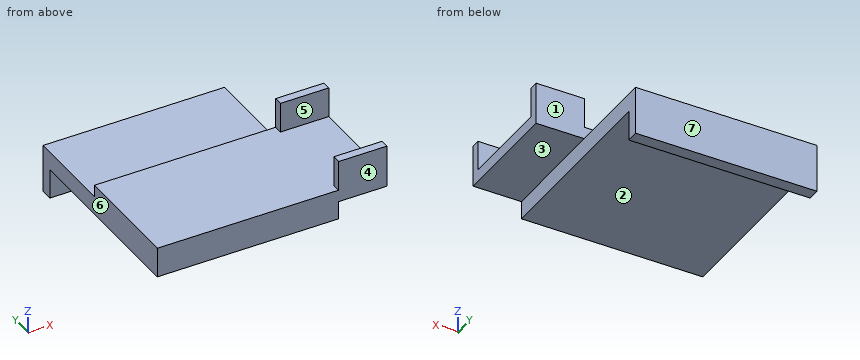
```python
from build123d import *

# Parameters (mm, degrees)
SKETCH2_W           = 50.8
SKETCH2_H           = 23.368
BOSS_EXTRUDE1_DEPTH = 2.54
SKETCH3_W           = 12.7
SKETCH3_H           = 1.778
BOSS_EXTRUDE2_DEPTH = 6.35
SKETCH4_W           = 2.54
SKETCH4_H           = 8.89
CUT_EXTRUDE1_DEPTH  = 24.368
BOSS_EXTRUDE3_DEPTH = 3.81
SKETCH10_W          = 38.1
SKETCH10_H          = 2.54
BOSS_EXTRUDE6_DEPTH = 6.35
SCALE1_SCALE        = 1.02


with BuildPart() as part:
    # Sketch2 → Boss-Extrude1 (new body)
    with BuildSketch(Plane.XY):
        Rectangle(SKETCH2_W, SKETCH2_H)
    extrude(amount=BOSS_EXTRUDE1_DEPTH)

    # Sketch3 → Boss-Extrude2 (add)
    with BuildSketch(Plane.XY.offset(2.54)):
        with Locations((19.05, 10.795)):
            Rectangle(SKETCH3_W, SKETCH3_H)
        with Locations((19.05, -10.795)):
            Rectangle(SKETCH3_W, SKETCH3_H)
    extrude(amount=BOSS_EXTRUDE2_DEPTH)

    # Sketch4 → Cut-Extrude1 (cut, through all)
    with BuildSketch(Plane(origin=(0, 11.684, 0), x_dir=(1, 0, 0), z_dir=(0, 1, 0))):
        with Locations((24.13, -4.445)):
            Rectangle(SKETCH4_W, SKETCH4_H)
    extrude(amount=-CUT_EXTRUDE1_DEPTH, mode=Mode.SUBTRACT)

    # Sketch5 → Boss-Extrude3 (add)
    with BuildSketch(Plane(origin=(0, 0, 0), x_dir=(-1, 0, 0), z_dir=(0, 0, -1))):
        Polygon((25.4, 11.684), (25.4, -11.684), (-12.7, -11.684), (-12.7, 11.684), (-12.7, 30.734), (25.4, 30.734), align=None)
    extrude(amount=BOSS_EXTRUDE3_DEPTH)

    # Sketch10 → Boss-Extrude6 (add)
    with BuildSketch(Plane(origin=(0, 0, -3.81), x_dir=(-1, 0, 0), z_dir=(0, 0, -1))):
        with Locations((6.35, 29.464)):
            Rectangle(SKETCH10_W, SKETCH10_H)
    extrude(amount=BOSS_EXTRUDE6_DEPTH)


with BuildPart() as part_1:
    # Scale1: scaled about (-4.313949838, 7.779949755, -1.122390582)
    add(part.part.scale(SCALE1_SCALE).moved(Location((0.086278997, -0.155598995, 0.022447812))))


solid = part_1.part
```
Can you work these out from the model? Positions are in its coordinate system, mm. Face numbers are marked on the shaded views. A direction names the side the tool comes from. Give positions to 0.01 mm unless a question says otherwise; leave off trailing zeros. Write each loop counter-clockwise with the first axis right and the second up, starting at its lowest first coordinate (ties: lowest second). Pieces come first, ordered by that corner, then holes. Notation, with made-up numbers: (80.5, -32) -> (129.5, -32) arc R30 cw to (129.5, 1) -> close; hole circle Ø4 at (76, 36.25). An arc over 180 degrees is marked (long way). One line per item, written item: value.
Q1. Imagine slicing it at B-B on x = 14.5. Please give me the cut outline in (y, z).
Results found:
outline: (-12.07, 0.02) -> (11.76, 0.02) -> (11.76, 9.09) -> (9.95, 9.09) -> (9.95, 2.61) -> (-10.26, 2.61) -> (-10.26, 9.09) -> (-12.07, 9.09) -> close
Q2. Please list where these lines run through material, in increasing order: line 1 (Z direction, x = 12.5, y = -2); line 2 (X direction, y = 29, z = -4.75); line 3 (Y direction, x = 9, z = -8.75). Write a range as [from, to].
Results found:
line 1: z = [-3.86, 2.61]
line 2: x = [-25.82, 13.04]
line 3: y = [28.6, 31.19]
Q3. We'd pull the mould along Y, two halves only. Please class the marked faces 5, 6 and 7: +Y half, -Y half, draft (parallel to the pull), parting line (faces both ways), or undercut.
Results found:
face 5: undercut
face 6: draft
face 7: +Y half
Q4. Which directions (+Z, -Z, +X, -X, +Y, -Y) give clear straight access to the entire face, cutting with the end or side of a thin tool? Please do the marked faces 1, 2, 3 and 4.
Results found:
face 1: +Z, +X, -X, +Y
face 2: -Z, +X, -X, -Y
face 3: -Z, +X, +Y, -Y
face 4: +Z, -Z, +X, -X, -Y
Q5. Imagine slicing it at D-D on z = -1. Please give me the cut outline in (x, y), and give its area (3 significant figures).
Results found:
outline: (-25.82, -12.07) -> (13.04, -12.07) -> (13.04, 31.19) -> (-25.82, 31.19) -> close
area: 1,680 mm^2
Q6. Imagine slicing it at A-A on z = 5.25. Please give me the cut outline in (x, y), and give its area (3 significant figures).
Results found:
outline: (13.04, -12.07) -> (23.4, -12.07) -> (23.4, -10.26) -> (13.04, -10.26) -> close; (13.04, 9.95) -> (23.4, 9.95) -> (23.4, 11.76) -> (13.04, 11.76) -> close
area: 37.6 mm^2
Q7. Imagine slicing it at C-C on y = -2.5. Please give me the cut outline in (x, z), and give its area (3 significant figures).
Results found:
outline: (-25.82, -3.86) -> (13.04, -3.86) -> (13.04, 0.02) -> (23.4, 0.02) -> (23.4, 2.61) -> (-25.82, 2.61) -> close
area: 279 mm^2
Q8. For P1, Ø11.5, axis at x = 18, y = 4, coming from the -Z side; P2, Ø5, axis at x = -16.5, z = 6, coming from the +Y side; P3, Ø6, axis at x = 8.5, y = 11.5, coming from the +Z side; P4, Ø0.9, axis at y = -11, z = 7.5, coming from the -X side, each with a flat end and sliding along its axis, tell me the tip position at first contact or that it passes through.
Results found:
P1: stops at z = -3.86
P2: passes through
P3: stops at z = 2.61
P4: stops at x = 13.04
